Source: CAD feature listing. Evaluate the final solid. Frame: model axes, mm. Face numbers are marked on the shaded views. Give positions to 0.01 mm unless a question says otherwise; leave off trailing zeros. Loops run counter-clockwise (first coordinate to the right, second up) from the corner with the lowest first, then second, coordinate; pieces in that order, holes last. Notation, with made-up numbers: (55, 37) -> (79, 37) arc R18 ccw to (79, 41) -> close; hole circle Ø10 at (-10, 25). An arc over 180 degrees is marked (long way). Answer as a JSON object with one key per item and string values. Group by question number.
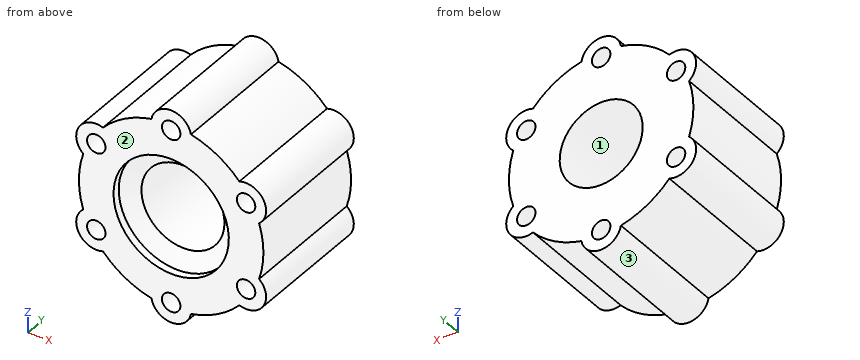
from build123d import *

# Parameters (mm, degrees)
SKETCH1_R           = 2.54
SKETCH1_R_2         = 15.875
BOSS_EXTRUDE1_DEPTH = 4.699
SKETCH2_R           = 11.426
SKETCH2_R_2         = 2.54
BOSS_EXTRUDE2_DEPTH = 30.301


with BuildPart() as part:
    # Sketch1 → Boss-Extrude1 (new body)
    with BuildSketch(Plane(origin=(0, 0, 0), x_dir=(1, 0, 0), z_dir=(0, 1, 0))):
        with BuildLine():
            ThreePointArc((-5.433318575, 24.812074667), (-12.7, 21.997045256), (-18.771227695, 17.111429246))
            ThreePointArc((-18.771227695, 17.111429246), (-25.406587271, 14.6685), (-24.204546269, 7.700645421))
            ThreePointArc((-24.204546269, 7.700645421), (-25.4, 0), (-24.204546269, -7.700645421))
            ThreePointArc((-24.204546269, -7.700645421), (-25.406587271, -14.6685), (-18.771227695, -17.111429246))
            ThreePointArc((-18.771227695, -17.111429246), (-12.7, -21.997045256), (-5.433318575, -24.812074667))
            ThreePointArc((-5.433318575, -24.812074667), (0, -29.337), (5.433318575, -24.812074667))
            ThreePointArc((5.433318575, -24.812074667), (12.7, -21.997045256), (18.771227695, -17.111429246))
            ThreePointArc((18.771227695, -17.111429246), (25.406587271, -14.6685), (24.204546269, -7.700645421))
            ThreePointArc((24.204546269, -7.700645421), (25.4, 0), (24.204546269, 7.700645421))
            ThreePointArc((24.204546269, 7.700645421), (25.406587271, 14.6685), (18.771227695, 17.111429246))
            ThreePointArc((18.771227695, 17.111429246), (12.7, 21.997045256), (5.433318575, 24.812074667))
            ThreePointArc((5.433318575, 24.812074667), (0, 29.337), (-5.433318575, 24.812074667))
        make_face()
        with Locations(Location((0, 23.8125, 0), (0, 0, 270))):
            Circle(SKETCH1_R, mode=Mode.SUBTRACT)
        with Locations(Location((20.622229928, 11.90625, 0), (0, 0, 270))):
            Circle(SKETCH1_R, mode=Mode.SUBTRACT)
        with Locations(Location((20.622229928, -11.90625, 0), (0, 0, 270))):
            Circle(SKETCH1_R, mode=Mode.SUBTRACT)
        with Locations(Location((0, -23.8125, 0), (0, 0, 270))):
            Circle(SKETCH1_R, mode=Mode.SUBTRACT)
        with Locations(Location((-20.622229928, -11.90625, 0), (0, 0, 270))):
            Circle(SKETCH1_R, mode=Mode.SUBTRACT)
        with Locations(Location((-20.622229928, 11.90625, 0), (0, 0, 270))):
            Circle(SKETCH1_R, mode=Mode.SUBTRACT)
        with Locations(Location((0, 0, 0), (0, 0, 270))):
            Circle(SKETCH1_R_2, mode=Mode.SUBTRACT)
    extrude(amount=BOSS_EXTRUDE1_DEPTH)

    # Sketch2 → Boss-Extrude2 (add)
    with BuildSketch(Plane(origin=(0, 4.699, 0), x_dir=(1, 0, 0), z_dir=(0, 1, 0))):
        with BuildLine():
            ThreePointArc((-18.771227695, 17.111429246), (-25.406587271, 14.6685), (-24.204546269, 7.700645421))
            ThreePointArc((-24.204546269, 7.700645421), (-25.4, 0), (-24.204546269, -7.700645421))
            ThreePointArc((-24.204546269, -7.700645421), (-25.406587271, -14.6685), (-18.771227695, -17.111429246))
            ThreePointArc((-18.771227695, -17.111429246), (-12.7, -21.997045256), (-5.433318575, -24.812074667))
            ThreePointArc((-5.433318575, -24.812074667), (0, -29.337), (5.433318575, -24.812074667))
            ThreePointArc((5.433318575, -24.812074667), (12.7, -21.997045256), (18.771227695, -17.111429246))
            ThreePointArc((18.771227695, -17.111429246), (25.406587271, -14.6685), (24.204546269, -7.700645421))
            ThreePointArc((24.204546269, -7.700645421), (25.4, 0), (24.204546269, 7.700645421))
            ThreePointArc((24.204546269, 7.700645421), (25.406587271, 14.6685), (18.771227695, 17.111429246))
            ThreePointArc((18.771227695, 17.111429246), (12.7, 21.997045256), (5.433318575, 24.812074667))
            ThreePointArc((5.433318575, 24.812074667), (0, 29.337), (-5.433318575, 24.812074667))
            ThreePointArc((-5.433318575, 24.812074667), (-12.7, 21.997045256), (-18.771227695, 17.111429246))
        make_face()
        with Locations(Location((0, 0, 0), (0, 0, 90))):
            Circle(SKETCH2_R, mode=Mode.SUBTRACT)
        with Locations(Location((20.622229928, -11.90625, 0), (0, 0, 90))):
            Circle(SKETCH2_R_2, mode=Mode.SUBTRACT)
        with Locations(Location((20.622229928, 11.90625, 0), (0, 0, 90))):
            Circle(SKETCH2_R_2, mode=Mode.SUBTRACT)
        with Locations(Location((0, 23.8125, 0), (0, 0, 90))):
            Circle(SKETCH2_R_2, mode=Mode.SUBTRACT)
        with Locations(Location((-20.622229928, 11.90625, 0), (0, 0, 90))):
            Circle(SKETCH2_R_2, mode=Mode.SUBTRACT)
        with Locations(Location((-20.622229928, -11.90625, 0), (0, 0, 90))):
            Circle(SKETCH2_R_2, mode=Mode.SUBTRACT)
        with Locations(Location((0, -23.8125, 0), (0, 0, 90))):
            Circle(SKETCH2_R_2, mode=Mode.SUBTRACT)
    extrude(amount=BOSS_EXTRUDE2_DEPTH)

    # Sketch3 → Revolve1 (revolve)
    with BuildSketch(Plane.XY, mode=Mode.PRIVATE) as revolve1_sk:
        Polygon((18.415, 2.0748), (18.415, 4.699), (11.426, 4.699), (15.875, 2.0748), align=None)
    revolve(revolve1_sk.sketch.rotate(Axis((0, -0.263075, 0), (0, 1, 0)), 90), axis=Axis((0, -0.263075, 0), (0, 1, 0)))


solid = part.part
(1) Section query A-A on x = 0. Return the cut outline in (y, z) (1 decimal).
(2) First-contact query: pin 1 (12 mm diameter, centred on x = -9, z = -2, fed in from -Y); pin 2 (4 mm diameter, centred on x = 20.62, z = -11.91, fed in from -Y); pin 3 (8 mm diameter, centred on x = 8, y = 6, fed in from +Z); pin 4 (1 mm diameter, centred on y = 30, z = -4, fed in from +X). Flat tips, straight axial feed; report the tip coordinate or a pass-through.
(3) Material intervals for line 1 (X direction, y = 9, z = 12); line 2 (X direction, y = 17, z = 0); line 3 (Z direction, x = -0.5, y = 14.5), sorted ascending. Write a range as from..to.
(4) Section query C-C on y = 10. Return the cut outline in (x, z), plus the area to 3 significant figures.
(5) Mould query, pull axis X, two halves, no side actions, for the marked faces 1, 2 and 3. Classes: pulls with the +X half, pulls with the -X half, needs draft (parallel to the pull), parting line crosses it, or undercut.
(6) Section query B-B on z = 0. Return the cut outline in (x, y) (3 decimals), plus the area to 3 significant figures.
Result:
{
 "1": {"outline": "(0, -29.3) -> (35, -29.3) -> (35, -26.4) -> (0, -26.4) -> close; (0, -21.3) -> (35, -21.3) -> (35, -11.4) -> (4.7, -11.4) -> (2.1, -15.9) -> (0, -15.9) -> close; (0, 15.9) -> (2.1, 15.9) -> (4.7, 11.4) -> (35, 11.4) -> (35, 21.3) -> (0, 21.3) -> close; (0, 26.4) -> (35, 26.4) -> (35, 29.3) -> (0, 29.3) -> close"},
 "2": {"pin 1": "y = 2.46", "pin 2": "through", "pin 3": "z = 27.62", "pin 4": "x = 25.16"},
 "3": {"line 1": "-26.15..-23.16, -18.08..18.08, 23.16..26.15", "line 2": "-25.4..-11.43, 11.43..25.4", "line 3": "-29.31..-26.3, -21.32..-11.42, 11.42..21.32, 26.3..29.31"},
 "4": {"outline": "(-24.2, -7.7) arc R5.52 ccw to (-18.77, -17.11) arc R25.4 ccw to (-5.43, -24.81) arc R5.52 ccw to (5.43, -24.81) arc R25.4 ccw to (18.77, -17.11) arc R5.52 ccw to (24.2, -7.7) arc R25.4 ccw to (24.2, 7.7) arc R5.52 ccw to (18.77, 17.11) arc R25.4 ccw to (5.43, 24.81) arc R5.52 ccw to (-5.43, 24.81) arc R25.4 ccw to (-18.77, 17.11) arc R5.52 ccw to (-24.2, 7.7) arc R25.4 ccw to start; hole circle Ø5.08 at (-20.62, -11.91); hole circle Ø5.08 at (-20.62, 11.91); hole circle Ø22.85 at (0, 0); hole circle Ø5.08 at (0, -23.81); hole circle Ø5.08 at (0, 23.81); hole circle Ø5.08 at (20.62, -11.91); hole circle Ø5.08 at (20.62, 11.91)", "area": "1,690 mm²"},
 "5": {"face 1": "undercut", "face 2": "needs draft", "face 3": "parting line crosses it"},
 "6": {"outline": "(-25.4, 0) -> (-15.875, 0) -> (-15.875, 2.075) -> (-11.426, 4.699) -> (-11.426, 35) -> (-25.4, 35) -> close; (11.426, 4.699) -> (15.875, 2.075) -> (15.875, 0) -> (25.4, 0) -> (25.4, 35) -> (11.426, 35) -> close", "area": "948 mm²"}
}
